Geometry: final body of the model. Coordinates: model frame, mm. Face numbers are marked on the shaded views. A direction names the side the tool comes from. Give positions to 0.01 mm unless a question says otherwise; leave off trailing zeros. Write each loop counter-clockwise with the first axis right and the second up, starting at its lowest first coordinate (ties: lowest second). Pieces come first, ordered by that corner, then holes.
Q1. Cut plane C-C on y = 82. Return the cut outline in (x, z).
Q2. Cut plane D-D on x = 25. Return the cut outline in (y, z), plus the area to 3 significant figures.
Q3. Reachability of the marked faces 1, 2, 3 and 4 from +Z, -Z, +X, -X, +Y, -Y: full face, straight path, thin tool, end or side. Return the list, or none.
Q4. Cut plane B-B on x = 13. Return the cut outline in (y, z), plus the area to 3 significant figures.
Q5. Pin query (flat end, axial travel): pin 1 (2 mm diameter, centred on x = 21, y = 83.5, fed in from +Z); pin 2 (10 mm diameter, centred on y = 33.5, z = 20, fed in from -X); pin 3 (9.5 mm diameter, centred on x = 26, z = -8, fed in from -Y); pin 4 (5 mm diameter, centred on y = 18, z = -4.5, fed in from -X). Return the tip coordinate at first contact, or that it passes through.
Q6. Draft query along X for the marked faces 5, 6 and 7. Return one class per face: pulls with the +X half, pulls with the -X half, needs draft (parallel to the pull), parting line crosses it, or undercut.
Q7. Cut plane A-A on z = -1. Return the cut outline in (x, y), plus the area to 3 significant figures.
Q8. Line query: L1, parallel to Y at x = 37, z = -2; L2, parallel to X at y = 82, z = -2; L3, parallel to Y at x = 32.5, z = 5.5. Output: solid intervals per line, ascending.
```python
from build123d import *

# Parameters (mm, degrees)
SKETCH1_W               = 50
SKETCH1_H               = 100
BOSS_EXTRUDE1_DEPTH     = 30
SKETCH2_W               = 42
SKETCH2_H               = 92
CUT_EXTRUDE1_DEPTH      = 26
SKETCH3_W               = 30
SKETCH3_H               = 6
BOSS_EXTRUDE2_DEPTH     = 24
CUT_EXTRUDE2_DEPTH      = 104.07764064
CUT_EXTRUDE2_DEPTH_BACK = 104.07764064
SKETCH4_R               = 9
CUT_EXTRUDE3_DEPTH      = 125.161185561
CUT_EXTRUDE3_DEPTH_BACK = 125.161185561
SKETCH5_R               = 1.5
CUT_EXTRUDE4_DEPTH      = 104.07764064
CUT_EXTRUDE4_DEPTH_BACK = 104.07764064
SKETCH6_W               = 30
SKETCH6_H               = 12


with BuildPart() as part:
    # Sketch1 → Boss-Extrude1 (new body)
    with BuildSketch(Plane.XY):
        with Locations((25, 50)):
            Rectangle(SKETCH1_W, SKETCH1_H)
    extrude(amount=BOSS_EXTRUDE1_DEPTH)

    # Sketch2 → Cut-Extrude1 (cut)
    with BuildSketch(Plane.XY.offset(30)):
        with Locations((25, 50)):
            Rectangle(SKETCH2_W, SKETCH2_H)
    extrude(amount=-CUT_EXTRUDE1_DEPTH, mode=Mode.SUBTRACT)

    # Sketch3 → Boss-Extrude2 (add)
    with BuildSketch(Plane(origin=(0, 0, 0), x_dir=(-1, 0, 0), z_dir=(0, 0, -1))):
        with Locations((-25, 18)):
            Rectangle(SKETCH3_W, SKETCH3_H)
        with Locations((-25, 82)):
            Rectangle(SKETCH3_W, SKETCH3_H)
    extrude(amount=BOSS_EXTRUDE2_DEPTH)

    # Sketch4 → Cut-Extrude2 (cut, two sides: drawn at the far end of the back side and taken through both)
    with BuildSketch(Plane.XZ.offset(-15).offset(-CUT_EXTRUDE2_DEPTH_BACK)):
        with Locations((25, -12)):
            Circle(SKETCH4_R)
    extrude(amount=CUT_EXTRUDE2_DEPTH + CUT_EXTRUDE2_DEPTH_BACK, mode=Mode.SUBTRACT)

    # Sketch5 → Cut-Extrude3 (cut, two sides: drawn at the far end of the back side and taken through both)
    with BuildSketch(Plane(origin=(0, 0, -24), x_dir=(-1, 0, 0), z_dir=(0, 0, -1)).offset(-CUT_EXTRUDE3_DEPTH_BACK)):
        with Locations((-13, 18)):
            Circle(SKETCH5_R)
        with Locations((-37, 18)):
            Circle(SKETCH5_R)
        with Locations((-13, 82)):
            Circle(SKETCH5_R)
        with Locations((-37, 82)):
            Circle(SKETCH5_R)
    extrude(amount=CUT_EXTRUDE3_DEPTH + CUT_EXTRUDE3_DEPTH_BACK, mode=Mode.SUBTRACT)

    # Sketch6 → Cut-Extrude4 (cut, two sides: drawn at the far end of the back side and taken through both)
    with BuildSketch(Plane.XZ.offset(-15).offset(-CUT_EXTRUDE4_DEPTH_BACK)):
        with Locations((25, -18)):
            Rectangle(SKETCH6_W, SKETCH6_H)
    extrude(amount=CUT_EXTRUDE4_DEPTH + CUT_EXTRUDE4_DEPTH_BACK, mode=Mode.SUBTRACT)


solid = part.part
```
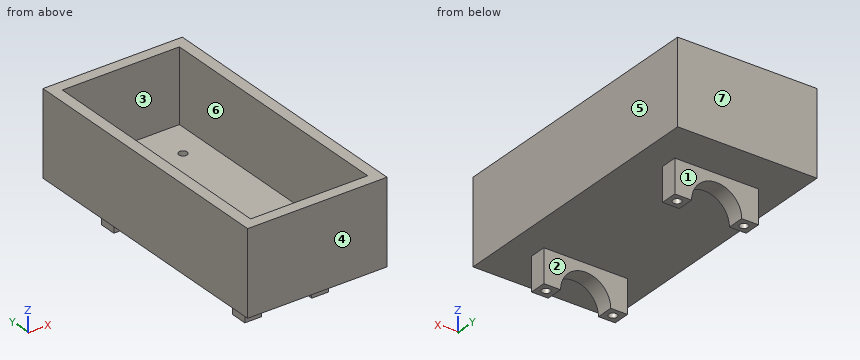
Data:
1. outline: (0, 0) - (10, 0) - (10, -12) - (11.5, -12) - (11.5, 4) - (4, 4) - (4, 30) - (0, 30) - close; (14.5, -12) - (16, -12) arc R9 cw to (34, -12) - (35.5, -12) - (35.5, 4) - (14.5, 4) - close; (38.5, -12) - (40, -12) - (40, 0) - (50, 0) - (50, 30) - (46, 30) - (46, 4) - (38.5, 4) - close
2. outline: (0, 0) - (15, 0) - (15, -3) - (21, -3) - (21, 0) - (79, 0) - (79, -3) - (85, -3) - (85, 0) - (100, 0) - (100, 30) - (96, 30) - (96, 4) - (4, 4) - (4, 30) - (0, 30) - close
2. area: 644 mm2
3. face 1: -Z, +X, -X, +Y
3. face 2: -Z, +X, -X
3. face 3: +Z
3. face 4: +Z, -Z, +X, -X, -Y
4. outline: (0, 0) - (15, 0) - (15, -12) - (16.5, -12) - (16.5, 4) - (4, 4) - (4, 30) - (0, 30) - close; (19.5, -12) - (21, -12) - (21, 0) - (79, 0) - (79, -12) - (80.5, -12) - (80.5, 4) - (19.5, 4) - close; (83.5, -12) - (85, -12) - (85, 0) - (100, 0) - (100, 30) - (96, 30) - (96, 4) - (83.5, 4) - close
4. area: 656 mm2
5. pin 1: stops at z = 4
5. pin 2: stops at x = 0
5. pin 3: passes through
5. pin 4: stops at x = 10
6. face 5: pulls with the +X half
6. face 6: undercut
6. face 7: needs draft
7. outline: (10, 15) - (40, 15) - (40, 21) - (10, 21) - close; (10, 79) - (40, 79) - (40, 85) - (10, 85) - close; hole circle Ø3 at (13, 18); hole circle Ø3 at (13, 82); hole circle Ø3 at (37, 18); hole circle Ø3 at (37, 82)
7. area: 332 mm2
8. L1: y = 15 to 16.5, 19.5 to 21, 79 to 80.5, 83.5 to 85
8. L2: x = 10 to 11.5, 14.5 to 35.5, 38.5 to 40
8. L3: y = 0 to 4, 96 to 100
